Geometry check sheet. Reference: the model listing, model coordinates, mm. Face numbers are marked on the shaded views. A direction names the side the tool comes from. Coordinates: 2 decimals unless noted, no trailing zeros. Order: outer loops, then holes, each group sorted by start corner. A loop starts at its lowest first (then second) coordinate and runs counter-clockwise, first axis right, second up. Notation, with made-up numbers: M 87.5,88 L 123.5,88 A15 ccw 123.5,96 Z; hole C -24,-35 d7. An arc over 180 degrees is marked long. One line per item, written item: value. Start each with the question number.
1) Thickness scan on L1, parallel to Y at x = -35.5, z = 12; L2, parallel to Z at x = -37, y = -0.25; L3, parallel to Z at x = -36, y = -16.5. Record the ranges inside material, lowest first. Write a range as from..to.
2) Access from +Z, -Z, +X, -X, +Y, -Y to the whole of each face (thin tool, end or side, straight path). Record for the marked faces 1 and 2.
3) Sectioned sample at B-B, the plane y = -14.5. Enter the section's corners in (x, z).
4) Sectioned sample at A-A, the plane x = -37.5. Enter the section's corners in (y, z).
5) Go/stop test with flat-tipped pins: P1, Ø1, axis at y = -15.5, z = 11, coming from the -X side; P2, Ø1.5, axis at x = -38, y = -0.5, coming from the +Z side; P3, Ø1, axis at y = -9.5, z = 15.5, coming from the +X side. Record where each tip stops, or that it passes through.
6) Sectioned sample at C-C, the plane z = 41.5. Enter the section's corners in (x, y).
7) Sectioned sample at D-D, the plane x = -31. Enter the section's corners in (y, z).
```python
from build123d import *

# Parameters (mm, degrees)
F0_R     = 6
F1_DEPTH = 45
F0_R_2   = 8
F2_DEPTH = 26
F0_R_3   = 11
F3_DEPTH = 20


with BuildPart() as f1:
    # F0 (on Top) → F1 (new body)
    with BuildSketch(Plane.XY):
        with Locations((-35.2753475308, -8.006202057)):
            Circle(F0_R)
    extrude(amount=F1_DEPTH)

    # F0 (on Top) → F2 (join)
    with BuildSketch(Plane.XY):
        with Locations((-35.2753475308, -8.006202057)):
            Circle(F0_R_2)
        with Locations((-35.2753475308, -8.006202057)):
            Circle(F0_R, mode=Mode.SUBTRACT)
    extrude(amount=F2_DEPTH)

    # F0 (on Top) → F3 (join)
    with BuildSketch(Plane.XY):
        with Locations((-35.2753475308, -8.006202057)):
            Circle(F0_R_3)
        with Locations((-35.2753475308, -8.006202057)):
            Circle(F0_R_2, mode=Mode.SUBTRACT)
    extrude(amount=F3_DEPTH)


solid = f1.part
```
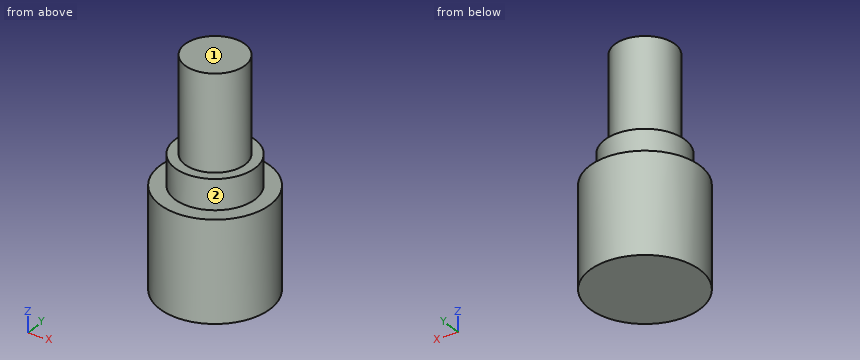
Final values:
1. L1: y = -19..2.99
1. L2: z = 0..26
1. L3: z = 0..20
2. face 1: +Z, +X, -X, +Y, -Y
2. face 2: +Z
3. outline: M -44.15,0 L -26.4,0 L -26.4,20 L -30.6,20 L -30.6,26 L -39.95,26 L -39.95,20 L -44.15,20 Z
4. outline: M -18.78,0 L 2.77,0 L 2.77,20 L -0.32,20 L -0.32,26 L -2.43,26 L -2.43,45 L -13.58,45 L -13.58,26 L -15.69,26 L -15.69,20 L -18.78,20 Z
5. P1: stops at x = -43.77
5. P2: stops at z = 26
5. P3: stops at x = -24.32
6. outline: C -35.28,-8.01 d12
7. outline: M -18.14,0 L 2.13,0 L 2.13,20 L -1.24,20 L -1.24,26 L -3.8,26 L -3.8,45 L -12.22,45 L -12.22,26 L -14.77,26 L -14.77,20 L -18.14,20 Z
